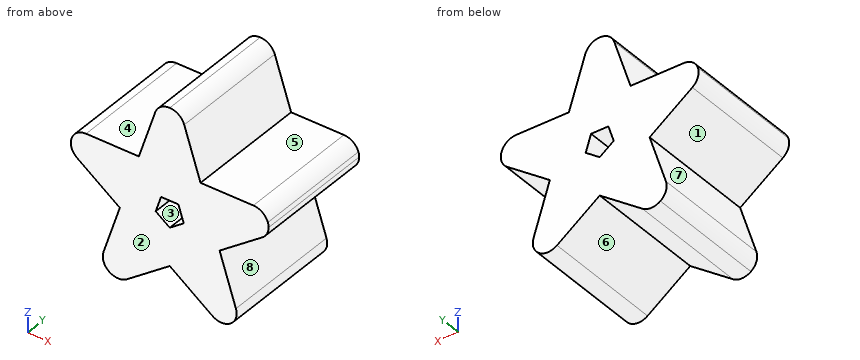
```python
from build123d import *

# Parameters (mm, degrees)
F1_DEPTH = 25.4
F2_DEPTH = 25.4
F3_DEPTH = 25.4
F4_DEPTH = 25.4
F5_DEPTH = 25.4


with BuildPart() as f1:
    # F0 (on Front) → F1 (new body)
    with BuildSketch(Plane.XZ):
        with BuildLine():
            ThreePointArc((3.0196044392, 17.3193664988), (3.1359104814, 17.8038160294), (3.175, 18.3004954559))
            ThreePointArc((3.175, 18.3004954559), (3.1359104814, 18.7971748824), (3.0196044392, 19.2816244131))
            ThreePointArc((3.0196044392, 19.2816244131), (1.8662181994, 20.8691243961), (5.78e-08, 21.4754954559))
            ThreePointArc((5.78e-08, 21.4754954559), (-1.866217236, 20.869125096), (-3.019603739, 19.2816265682))
            ThreePointArc((-3.019603739, 19.2816265682), (-3.175, 18.3004954559), (-3.019603739, 17.3193643436))
            ThreePointArc((-3.019603739, 17.3193643436), (1.133e-06, 15.1254954559), (3.0196044392, 17.3193664988))
        make_face()
        with BuildLine():
            Line((0.261295375, 8.8301641014), (3.0196044392, 17.3193664988))
            ThreePointArc((3.0196044392, 17.3193664988), (1.133e-06, 15.1254954559), (-3.019603739, 17.3193643436))
            Line((-3.019603739, 17.3193643436), (-0.261295375, 8.8301641014))
            Line((-0.261295375, 8.8301641014), (0.261295375, 8.8301641014))
        make_face()
        with BuildLine():
            Line((-0.261295375, 8.8301641014), (-3.019603739, 17.3193643436))
            ThreePointArc((-3.019603739, 17.3193643436), (-3.175, 18.3004954559), (-3.019603739, 19.2816265682))
            Line((-3.019603739, 19.2816265682), (-6.4154897489, 8.8301641014))
            Line((-6.4154897489, 8.8301641014), (-0.261295375, 8.8301641014))
        make_face()
        Polygon((0, 8.0259796274), (-0.261295375, 8.8301641014), (-6.4154897489, 8.8301641014), (-8.3172403971, 2.9771774395), (-7.6331602243, 2.4801641014), (-1.8019446961, 2.4801641014), align=None)
        Polygon((-2.9156077641, -0.947338389), (-1.8019446961, 2.4801641014), (-7.6331602243, 2.4801641014), align=None)
        Polygon((-4.7175524602, -6.493153915), (-2.9156077641, -0.947338389), (-7.6331602243, 2.4801641014), (-8.47872982, 2.4801641014), (-10.3804804682, -3.3728225605), (-5.401632633, -6.9901672532), align=None)
        with BuildLine():
            Line((-5.401632633, -6.9901672532), (-10.3804804682, -3.3728225605))
            Line((-10.3804804682, -3.3728225605), (-13.7763657779, -13.8242828722))
            ThreePointArc((-13.7763657779, -13.8242828722), (-13.3253902958, -12.9391936533), (-12.6229795147, -12.2367828722))
            Line((-12.6229795147, -12.2367828722), (-5.401632633, -6.9901672532))
        make_face()
        with BuildLine():
            Line((-4.9788478352, -7.297338389), (-5.401632633, -6.9901672532))
            Line((-5.401632633, -6.9901672532), (-12.6229795147, -12.2367828722))
            ThreePointArc((-12.6229795147, -12.2367828722), (-9.315341502, -11.976466115), (-7.5817613386, -14.8054118293))
            ThreePointArc((-7.5817613386, -14.8054118293), (-7.6208508572, -15.3020912558), (-7.7371568994, -15.7865407865))
            Line((-7.7371568994, -15.7865407865), (-4.9788478352, -7.297338389))
        make_face()
        with BuildLine():
            ThreePointArc((-13.7763657779, -13.8242828722), (-13.7763657849, -15.7865407647), (-12.6229795517, -17.3740407596))
            ThreePointArc((-12.6229795517, -17.3740407596), (-10.7567613615, -17.9804118293), (-8.8905431626, -17.3740407865))
            ThreePointArc((-8.8905431626, -17.3740407865), (-8.1881323815, -16.6716300054), (-7.7371568994, -15.7865407865))
            ThreePointArc((-7.7371568994, -15.7865407865), (-7.6208508572, -15.3020912558), (-7.5817613386, -14.8054118293))
            ThreePointArc((-7.5817613386, -14.8054118293), (-9.315341502, -11.976466115), (-12.6229795147, -12.2367828722))
            ThreePointArc((-12.6229795147, -12.2367828722), (-13.3253902958, -12.9391936533), (-13.7763657779, -13.8242828722))
        make_face()
        Polygon((0, 8.0259796274), (0.261295375, 8.8301641014), (-0.261295375, 8.8301641014), align=None)
        Polygon((-4.9788478352, -7.297338389), (-4.7175524602, -6.493153915), (-5.401632633, -6.9901672532), align=None)
        Polygon((-7.6331602243, 2.4801641014), (-8.3172403971, 2.9771774395), (-8.47872982, 2.4801641014), align=None)
    extrude(amount=F1_DEPTH)

    # F0 (on Front) → F2 (join)
    with BuildSketch(Plane.XZ):
        with BuildLine():
            ThreePointArc((-17.4048054548, 8.8301641014), (-19.2710239415, 8.2237928328), (-20.4244101314, 6.636292328))
            ThreePointArc((-20.4244101314, 6.636292328), (-20.4244097753, 4.674034779), (-19.2710236308, 3.0865351442))
            ThreePointArc((-19.2710236308, 3.0865351442), (-18.3859344119, 2.6355596621), (-17.4048054548, 2.4801641014))
            ThreePointArc((-17.4048054548, 2.4801641014), (-15.1597414245, 3.4101000711), (-14.2298054548, 5.6551641014))
            ThreePointArc((-14.2298054548, 5.6551641014), (-14.5758597405, 7.096583938), (-15.5385872788, 8.2237930585))
            ThreePointArc((-15.5385872788, 8.2237930585), (-16.4236764976, 8.6747685406), (-17.4048054548, 8.8301641014))
        make_face()
        with BuildLine():
            Line((-8.3172403971, 2.9771774395), (-6.4154897489, 8.8301641014))
            Line((-6.4154897489, 8.8301641014), (-17.4048054548, 8.8301641014))
            ThreePointArc((-17.4048054548, 8.8301641014), (-16.4236764976, 8.6747685406), (-15.5385872788, 8.2237930585))
            Line((-15.5385872788, 8.2237930585), (-8.3172403971, 2.9771774395))
        make_face()
        with BuildLine():
            Line((-8.47872982, 2.4801641014), (-8.3172403971, 2.9771774395))
            Line((-8.3172403971, 2.9771774395), (-15.5385872788, 8.2237930585))
            ThreePointArc((-15.5385872788, 8.2237930585), (-14.5758597405, 7.096583938), (-14.2298054548, 5.6551641014))
            ThreePointArc((-14.2298054548, 5.6551641014), (-15.1597414245, 3.4101000711), (-17.4048054548, 2.4801641014))
            Line((-17.4048054548, 2.4801641014), (-8.47872982, 2.4801641014))
        make_face()
        Polygon((1.8019446961, 2.4801641014), (0, 8.0259796274), (-1.8019446961, 2.4801641014), align=None)
        Polygon((8.3172403971, 2.9771774395), (6.4154897489, 8.8301641014), (0.261295375, 8.8301641014), (0, 8.0259796274), (1.8019446961, 2.4801641014), (7.6331602243, 2.4801641014), align=None)
        with BuildLine():
            Line((17.4048054548, 8.8301641014), (6.4154897489, 8.8301641014))
            Line((6.4154897489, 8.8301641014), (8.3172403971, 2.9771774395))
            Line((8.3172403971, 2.9771774395), (15.5385872788, 8.2237930585))
            ThreePointArc((15.5385872788, 8.2237930585), (16.4236764976, 8.6747685406), (17.4048054548, 8.8301641014))
        make_face()
        with BuildLine():
            Line((15.5385872788, 8.2237930585), (8.3172403971, 2.9771774395))
            Line((8.3172403971, 2.9771774395), (8.47872982, 2.4801641014))
            Line((8.47872982, 2.4801641014), (17.4048054548, 2.4801641014))
            ThreePointArc((17.4048054548, 2.4801641014), (14.3852010155, 4.6740351442), (15.5385872788, 8.2237930585))
        make_face()
        with BuildLine():
            ThreePointArc((20.4244101232, 6.6362923532), (19.2710239308, 8.2237928405), (17.4048054548, 8.8301641014))
            ThreePointArc((17.4048054548, 8.8301641014), (16.4236764976, 8.6747685406), (15.5385872788, 8.2237930585))
            ThreePointArc((15.5385872788, 8.2237930585), (14.3852010155, 4.6740351442), (17.4048054548, 2.4801641014))
            ThreePointArc((17.4048054548, 2.4801641014), (18.3859344119, 2.6355596621), (19.2710236308, 3.0865351442))
            ThreePointArc((19.2710236308, 3.0865351442), (20.2337511691, 4.2137442647), (20.5798054548, 5.6551641014))
            ThreePointArc((20.5798054548, 5.6551641014), (20.5407159942, 6.1518431616), (20.4244101232, 6.6362923532))
        make_face()
        Polygon((8.47872982, 2.4801641014), (8.3172403971, 2.9771774395), (7.6331602243, 2.4801641014), align=None)
    extrude(amount=F2_DEPTH)

    # F0 (on Front) → F3 (join)
    with BuildSketch(Plane.XZ):
        with BuildLine():
            ThreePointArc((3.0196044392, 19.2816244131), (3.1359104814, 18.7971748824), (3.175, 18.3004954559))
            ThreePointArc((3.175, 18.3004954559), (3.1359104814, 17.8038160294), (3.0196044392, 17.3193664988))
            Line((3.0196044392, 17.3193664988), (0.261295375, 8.8301641014))
            Line((0.261295375, 8.8301641014), (6.4154897489, 8.8301641014))
            Line((6.4154897489, 8.8301641014), (3.0196044392, 19.2816244131))
        make_face()
        Polygon((2.9156077641, -0.947338389), (7.6331602243, 2.4801641014), (1.8019446961, 2.4801641014), align=None)
        Polygon((10.3804804682, -3.3728225605), (8.47872982, 2.4801641014), (7.6331602243, 2.4801641014), (2.9156077641, -0.947338389), (4.7175524602, -6.493153915), (5.401632633, -6.9901672532), align=None)
        with BuildLine():
            Line((13.7763657779, -13.8242828722), (10.3804804682, -3.3728225605))
            Line((10.3804804682, -3.3728225605), (5.401632633, -6.9901672532))
            Line((5.401632633, -6.9901672532), (12.6229795147, -12.2367828722))
            ThreePointArc((12.6229795147, -12.2367828722), (13.3253902958, -12.9391936533), (13.7763657779, -13.8242828722))
        make_face()
        with BuildLine():
            Line((12.6229795147, -12.2367828722), (5.401632633, -6.9901672532))
            Line((5.401632633, -6.9901672532), (4.9788478352, -7.297338389))
            Line((4.9788478352, -7.297338389), (7.7371568994, -15.7865407865))
            ThreePointArc((7.7371568994, -15.7865407865), (8.8905431626, -12.2367828722), (12.6229795147, -12.2367828722))
        make_face()
        with BuildLine():
            ThreePointArc((8.8905431626, -17.3740407865), (10.7567613452, -17.9804118293), (12.6229795253, -17.3740407787))
            ThreePointArc((12.6229795253, -17.3740407787), (13.5857070559, -16.2468316601), (13.9317613386, -14.8054118293))
            ThreePointArc((13.9317613386, -14.8054118293), (13.89267182, -14.3087324028), (13.7763657779, -13.8242828722))
            ThreePointArc((13.7763657779, -13.8242828722), (13.3253902958, -12.9391936533), (12.6229795147, -12.2367828722))
            ThreePointArc((12.6229795147, -12.2367828722), (8.8905431626, -12.2367828722), (7.7371568994, -15.7865407865))
            ThreePointArc((7.7371568994, -15.7865407865), (8.1881323815, -16.6716300054), (8.8905431626, -17.3740407865))
        make_face()
        Polygon((4.9788478352, -7.297338389), (5.401632633, -6.9901672532), (4.7175524602, -6.493153915), align=None)
    extrude(amount=F3_DEPTH)

    # F0 (on Front) → F4 (join)
    with BuildSketch(Plane.XZ):
        with BuildLine():
            ThreePointArc((-7.7371568994, -15.7865407865), (-8.1881323815, -16.6716300054), (-8.8905431626, -17.3740407865))
            Line((-8.8905431626, -17.3740407865), (0, -10.9146830818))
            Line((0, -10.9146830818), (-4.9788478352, -7.297338389))
            Line((-4.9788478352, -7.297338389), (-7.7371568994, -15.7865407865))
        make_face()
        Polygon((4.9788478352, -7.297338389), (4.7175524602, -6.493153915), (0, -3.0656514246), (-4.7175524602, -6.493153915), (-4.9788478352, -7.297338389), (0, -10.9146830818), align=None)
        Polygon((4.7175524602, -6.493153915), (2.9156077641, -0.947338389), (0, -3.0656514246), align=None)
        with BuildLine():
            Line((17.4048054548, 2.4801641014), (8.47872982, 2.4801641014))
            Line((8.47872982, 2.4801641014), (10.3804804682, -3.3728225605))
            Line((10.3804804682, -3.3728225605), (19.2710236308, 3.0865351442))
            ThreePointArc((19.2710236308, 3.0865351442), (18.3859344119, 2.6355596621), (17.4048054548, 2.4801641014))
        make_face()
    extrude(amount=F4_DEPTH)

    # F0 (on Front) → F5 (join)
    with BuildSketch(Plane.XZ):
        with BuildLine():
            ThreePointArc((-17.4048054548, 2.4801641014), (-18.3859344119, 2.6355596621), (-19.2710236308, 3.0865351442))
            Line((-19.2710236308, 3.0865351442), (-10.3804804682, -3.3728225605))
            Line((-10.3804804682, -3.3728225605), (-8.47872982, 2.4801641014))
            Line((-8.47872982, 2.4801641014), (-17.4048054548, 2.4801641014))
        make_face()
        Polygon((0, -3.0656514246), (-2.9156077641, -0.947338389), (-4.7175524602, -6.493153915), align=None)
        with BuildLine():
            Line((0, -10.9146830818), (8.8905431626, -17.3740407865))
            ThreePointArc((8.8905431626, -17.3740407865), (8.1881323815, -16.6716300054), (7.7371568994, -15.7865407865))
            Line((7.7371568994, -15.7865407865), (4.9788478352, -7.297338389))
            Line((4.9788478352, -7.297338389), (0, -10.9146830818))
        make_face()
    extrude(amount=F5_DEPTH)


solid = f1.part
```
CAD build for the part. Positions are in the model's coordinates, mm. Face numbers are marked on the shaded views. A direction names the side the tool comes from. Give positions to 0.01 mm unless a question says otherwise; leave off trailing zeros. Order: outer loops, then holes, each group sorted by start corner. A loop starts at its lowest first (then second) coordinate and runs counter-clockwise, first axis right, second up.
(1) Mould opens along X. For the marked faces 1, 2 and 3 say: released by +X, released by -X, zero draft, split by the parting line, or undercut.
(2) Saw through at C-C, the plane x = -8. Give the cut face in (y, z).
(3) Tool access for the marked faces 4, 5, 6, 7 and 8: list every direction of +Z, -Z, +X, -X, +Y, -Y with a clear straight run to the whole face (end or side of a thin tool).
(4) Flat gauge pins, fed straight in: pin 1 (8 mm diameter, centred on x = 14, z = 6, fed in from +Y); pin 2 (4 mm diameter, centred on y = -11.5, z = -7, fed in from +X); pin 3 (9 mm diameter, centred on x = -12.5, y = -15, fed in from +Z); pin 4 (3 mm diameter, centred on x = 0.5, y = -10, fed in from -Z). Where does each tip first touch, or does it go through?
(5) Drill centre lines: L1, parallel to Z at x = -1.5, y = -20; L2, parallel to X at y = -9, z = -15; L3, parallel to Z at x = 0.5, y = -5. Where is each one in solid material? Low to high.
(6) Saw through at B-B, the plane z = 15.5. Give the cut face in (x, y), then the cut area to 3 significant figures.
Results found:
1. face 1: released by -X
1. face 2: zero draft
1. face 3: undercut
2. outline: (-25.4, -16.73) - (0, -16.73) - (0, 8.83) - (-25.4, 8.83) - close
3. face 4: +Z, -X, +Y, -Y
3. face 5: +Z, +X, +Y, -Y
3. face 6: -Z, +Y, -Y
3. face 7: -X, +Y, -Y
3. face 8: +X, +Y, -Y
4. pin 1: stops at y = 0
4. pin 2: stops at x = 12.21
4. pin 3: stops at z = 8.83
4. pin 4: stops at z = -12.37
5. L1: z = -12 to -1.98, 2.48 to 21.1
5. L2: x = -13.93 to -5.62, 5.62 to 13.93
5. L3: z = -11.28 to -2.7, 2.48 to 21.44
6. outline: (-4.25, -25.4) - (4.25, -25.4) - (4.25, 0) - (-4.25, 0) - close
6. area: 216 mm2
